Could you check a few things on this model? Use its own coordinates, in mm. Face numbers are marked on the shaded views. Give positions to 0.01 mm unless a question says otherwise; leave off trailing zeros. Order: outer loops, then holes, each group sorted by start corner. A loop starts at its lowest first (then second) coordinate and runs counter-clockwise, first axis right, second up. Notation, with made-up numbers: M -8.5,88.25 L 9.5,88.25 A29 ccw 9.5,112.25 Z; hole C -30,27 d8. An arc over 180 degrees is marked long. Use a Markdown table: item, result. Add a question column.
Item 1: Suppose I cut it at A-A on x = 0. Write out the boundary of the cut face in (y, z), plus the area to 3 significant figures.
Item 2: If I drill on L1, parallel to X at y = 0, z = 23; L2, parallel to Z at x = -6.5, y = -17.5, over which ranges is the centre line in solid material (lowest first)? Write a range as from..to.
Item 3: If we mould it in two halves opening along X, with no side actions, what happens to the marked faces 1, 2 and 3? For each: released by +X, released by -X, zero draft, split by the parting line, or undercut.
Item 4: I'm going to push flat-ended pins straight in: pin 1 Ø2 at (y, z) = (-12.5, 99.5) entering from -X; pin 2 Ø8 at (y, z) = (-1, 54) entering from +X; pin 3 Ø4 at (x, z) = (-4.5, 15) entering from -Y (3 decimals). Where does each tip first touch, or does it pass through?
Item 5: Suppose I cut it at C-C on z = 30. Write out the boundary of the cut face in (x, y).
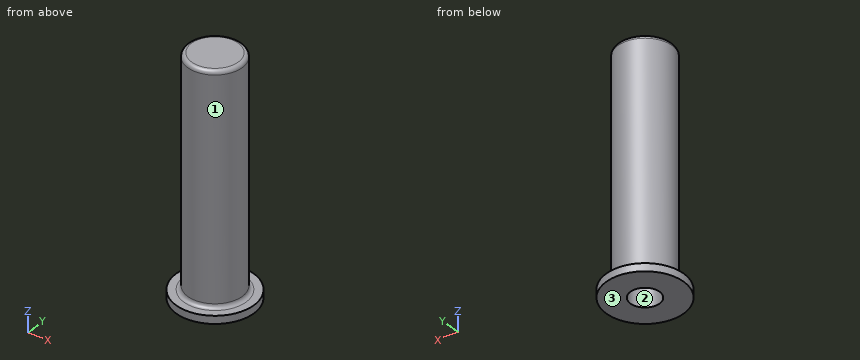
from build123d import *

# Parameters (mm, degrees)
SKETCH1_R           = 14
SKETCH1_R_2         = 7.5
BOSS_EXTRUDE1_DEPTH = 120
BOSS_EXTRUDE2_START = -10
SKETCH2_R           = 14
BOSS_EXTRUDE2_DEPTH = 10
SKETCH3_R           = 20
SKETCH3_R_2         = 7.5
BOSS_EXTRUDE3_DEPTH = 4
FILLET3_R           = 2


with BuildPart() as part:
    # Sketch1 → Boss-Extrude1 (new body)
    with BuildSketch(Plane.XY):
        Circle(SKETCH1_R)
        Circle(SKETCH1_R_2, mode=Mode.SUBTRACT)
    extrude(amount=BOSS_EXTRUDE1_DEPTH)

    # Sketch2 → Boss-Extrude2 (add)
    with BuildSketch(Plane.XY.offset(120).offset(BOSS_EXTRUDE2_START)):
        Circle(SKETCH2_R)
    extrude(amount=BOSS_EXTRUDE2_DEPTH)

    # Sketch3 → Boss-Extrude3 (add)
    with BuildSketch(Plane(origin=(0, 0, 0), x_dir=(-1, 0, 0), z_dir=(0, 0, -1))):
        Circle(SKETCH3_R)
        with Locations(Location((0, 0, 0), (0, 0, 180))):
            Circle(SKETCH3_R_2, mode=Mode.SUBTRACT)
    extrude(amount=-BOSS_EXTRUDE3_DEPTH)

    # Fillet3
    fillet3_edges = [part.edges().sort_by_distance(p)[0] for p in [
        (-14, 0, 4),
        (-14, 0, 120),
    ]]
    fillet(fillet3_edges, radius=FILLET3_R)


solid = part.part
Findings below:
| question | item | result |
|---|---|---|
| 1 | outline | M -20,0 L -7.5,0 L -7.5,110 L 7.5,110 L 7.5,0 L 20,0 L 20,4 L 16,4 A2 cw 14,6 L 14,118 A2 ccw 12,120 L -12,120 A2 ccw -14,118 L -14,6 A2 cw -16,4 L -20,4 Z |
| 1 | area | 1,760 mm^2 |
| 2 | L1 | x = -14..-7.5, 7.5..14 |
| 2 | L2 | z = 0..4 |
| 3 | face 1 | split by the parting line |
| 3 | face 2 | undercut |
| 3 | face 3 | zero draft |
| 4 | pin 1 | stops at x = -7.98 |
| 4 | pin 2 | stops at x = 14 |
| 4 | pin 3 | stops at y = -13.775 |
| 5 | outline | C 0,0 d28; hole C 0,0 d15 |
